from build123d import *

# Parameters (mm, degrees)
SKETCH3_R           = 24
SKETCH3_R_2         = 4
SKETCH3_R_3         = 3
BOSS_EXTRUDE1_DEPTH = 4


with BuildPart() as part:
    # Sketch1 → Revolve2 (revolve)
    with BuildSketch(Plane.XY, mode=Mode.PRIVATE) as revolve2_sk:
        Polygon((0, 24), (0, 34), (2, 34), (2, 30), (42, 30), (42, 34), (44, 34), (44, 24), align=None)
    revolve(revolve2_sk.sketch.rotate(Axis((0, 0, 0), (1, 0, 0)), 90), axis=Axis((0, 0, 0), (1, 0, 0)))

    # Sketch2 → Revolve3 (revolve)
    with BuildSketch(Plane.XY, mode=Mode.PRIVATE) as revolve3_sk:
        Polygon((2, 34), (2, 30), (42, 30), (42, 34), (42, 37), (2, 37), align=None)
    revolve(revolve3_sk.sketch.rotate(Axis((0, 0, 0), (1, 0, 0)), 90), axis=Axis((0, 0, 0), (1, 0, 0)))

    # Sketch3 → Boss-Extrude1 (add)
    with BuildSketch(Plane.ZY):
        Circle(SKETCH3_R)
        with Locations((19, 0)):
            Circle(SKETCH3_R_2, mode=Mode.SUBTRACT)
        Circle(SKETCH3_R_3, mode=Mode.SUBTRACT)
        with Locations((9.5, -16.454482672)):
            Circle(SKETCH3_R_2, mode=Mode.SUBTRACT)
        with Locations((-9.5, -16.454482672)):
            Circle(SKETCH3_R_2, mode=Mode.SUBTRACT)
        with Locations((-19, 0)):
            Circle(SKETCH3_R_2, mode=Mode.SUBTRACT)
        with Locations((-9.5, 16.454482672)):
            Circle(SKETCH3_R_2, mode=Mode.SUBTRACT)
        with Locations((9.5, 16.454482672)):
            Circle(SKETCH3_R_2, mode=Mode.SUBTRACT)
    extrude(amount=-BOSS_EXTRUDE1_DEPTH)


solid = part.part
For this review, take the finished solid that the model builds, in its own axes (mm). A direction names the side the tool comes from. Round coordinates to 2 decimals unless told otherwise and drop trailing zeros. Order: outer loops, then holes, each group sorted by start corner. A loop starts at its lowest first (then second) coordinate and runs counter-clockwise, first axis right, second up. Notation, with made-up numbers: M 20.5,-5.75 L 27.5,-5.75 A24 cw 27.5,21.25 Z; hole C 56.25,-16.5 d2. An arc over 180 degrees is marked long. Write each question's results on one line, items separated by ' | '. Start each with the question number.
1. Add section C-C (y = -14). State the section outline as (x, z) points, then the cut area to 3 significant figures.
2. To check wall thickness, follow L1, parallel to Y at x = 1.7, z = 9.5; L2, parallel to Y at x = 1, z = 0; L3, parallel to X at y = -11, z = -17.5. State the ranges of each line that lie inside material, in increasing order. Write a range as [from, to].
3. Draft analysis for pull direction Z (two halves, no side actions). For faces 4 (the face through (43.01, -33.71, -4.43)), 5 (the face through (2, -2.4, 15.8)), 6 (the face through (42, 33, -11)), state which applies: pulls with the +Z half, pulls with the -Z half, needs draft (parallel to the pull), parting line crosses it, or undercut.
4. Add section A-A (z = 0). State the section outline as (x, y) points, then the cut area to 3 significant figures.
5. Tool access review of faces 1 (the face through (1.972, 19.158, -12.448)), 2 (the face through (4, 0, 5)), 3 (the face through (2, 33, 11)): name each direction out of +Z, -Z, +X, -X, +Y, -Y from which nothing blocks a thin tool from reaching the whole face with its end or side.
6. Add section D-D (z = -8). State the section outline as (x, y) points, then the cut area to 3 significant figures.
7. Clearance check with flat-ended pins moving along their axes: pin 1 Ø12 at (x, z) = (15, 4) entering from -Y; pin 2 Ø6 at (y, z) = (11.5, -4) entering from +X; pin 3 Ø2 at (y, z) = (-26.5, 23) entering from -X. State where each tip first meets the part, or that it passes through.
8. Add section B-B (y = 0). State the section outline as (x, z) points.
Output values:
1) outline: M 0,-30.98 L 2,-30.98 L 2,-34.25 L 42,-34.25 L 42,-30.98 L 44,-30.98 L 44,-19.49 L 4,-19.49 L 4,-12.66 L 0,-12.66 Z; M 0,-6.34 L 4,-6.34 L 4,6.34 L 0,6.34 Z; M 0,12.66 L 4,12.66 L 4,19.49 L 44,19.49 L 44,30.98 L 42,30.98 L 42,34.25 L 2,34.25 L 2,30.98 L 0,30.98 Z | area: 1,380 mm^2
2) L1: [-32.65, -20.45], [-12.45, 12.45], [20.45, 32.65] | L2: [-34, -3], [3, 34] | L3: [0, 4]
3) face 4: parting line crosses it | face 5: undercut | face 6: needs draft
4) outline: M 0,-34 L 2,-34 L 2,-37 L 42,-37 L 42,-34 L 44,-34 L 44,-24 L 4,-24 L 4,-3 L 0,-3 Z; M 0,3 L 4,3 L 4,24 L 44,24 L 44,34 L 42,34 L 42,37 L 2,37 L 2,34 L 0,34 Z | area: 1,290 mm^2
5) face 1: +X, -X | face 2: +X | face 3: -X
6) outline: M 0,-33.05 L 2,-33.05 L 2,-36.12 L 42,-36.12 L 42,-33.05 L 44,-33.05 L 44,-22.63 L 4,-22.63 L 4,-20.16 L 0,-20.16 Z; M 0,-12.75 L 4,-12.75 L 4,12.75 L 0,12.75 Z; M 0,20.16 L 4,20.16 L 4,22.63 L 44,22.63 L 44,33.05 L 42,33.05 L 42,36.12 L 2,36.12 L 2,33.05 L 0,33.05 Z | area: 1,280 mm^2
7) pin 1: y = -37 | pin 2: x = 4 | pin 3: x = 2
8) outline: M 0,-34 L 2,-34 L 2,-37 L 42,-37 L 42,-34 L 44,-34 L 44,-24 L 4,-24 L 4,-23 L 0,-23 Z; M 0,-15 L 4,-15 L 4,-3 L 0,-3 Z; M 0,3 L 4,3 L 4,15 L 0,15 Z; M 0,23 L 4,23 L 4,24 L 44,24 L 44,34 L 42,34 L 42,37 L 2,37 L 2,34 L 0,34 Z
